Autodesk Inventor part; units mm, degrees
ref_plane "YZ Plane" through (0, 0, 0) normal (1, 0, 0) x (0, 1, 0)
ref_plane "XZ Plane" through (0, 0, 0) normal (0, 1, 0) x (-1, 0, 0)
ref_plane "XY Plane" through (0, 0, 0) normal (0, 0, 1) x (1, 0, 0)
sketch "Эскиз1" plane through (0, 0, 0) normal (0, 1, 0) x (-1, 0, 0)
  circle A0 centre (0, 0) radius 56
  circle A1 centre (46, 0) radius 5.5
  circle A2 centre (0, 46) radius 5.5
  circle A3 centre (-46, 0) radius 5.5
  circle A4 centre (0, -46) radius 5.5
  dimension "d0" = 112
  dimension "d1" = 11
  dimension "d2" = 46
  dimension "d5" = 360
extrude "Выдавливание1" add sketch "Эскиз1" along normal blind 10
sketch "Эскиз3" plane through (0, 10, 0) normal (0, 1, 0) x (1, 0, 0)
  circle A0 centre (0, 0) radius 22
  dimension "d9" = 44
extrude "Выдавливание2" cut sketch "Эскиз3" against normal blind 10
sketch "Эскиз4" plane through (0, 0, 0) normal (0, -1, 0) x (1, 0, 0)
  circle A0 centre (0, 0) radius 38
  dimension "d12" = 76
extrude "Выдавливание3" add sketch "Эскиз4" along normal blind 38
sketch "Эскиз5" plane through (0, -38, 0) normal (0, -1, 0) x (1, 0, 0)
  circle A0 centre (0, 0) radius 12.5
  dimension "d15" = 25
extrude "Выдавливание4" cut sketch "Эскиз5" against normal through all
chamfer "Фаска1" distance 1.6 angle 45 1 edges at (-22, 10, 0)
chamfer "Фаска2" distance 2.5 angle 45 1 edges at (-38, -38, 0)
sketch "Эскиз6" plane through (0, -38, 0) normal (0, -1, 0) x (1, 0, 0)
  point P0 (0, 0)
  point P1 (0, -24)
  point P2 (0, 24)
  dimension "d24" = 24
  dimension "d25" = 48
hole "Отверстие1" at (0, -38, -24) at (0, -38, 24) direction (0, 1, 0) diameter 8.376 depth 24 tip angle 120
chamfer "Фаска3" distance 1.6 angle 45 2 edges at (0, -38, -19.812) (0, -38, 28.188)
properties part number "Фланец"
CAD build for the part. Positions are in the model's coordinates, mm. A direction names the side the tool comes from. Give positions to 0.01 mm unless a question says otherwise; leave off trailing zeros. Order: outer loops, then holes, each group sorted by start corner. A loop starts at its lowest first (then second) coordinate and runs counter-clockwise, first axis right, second up. Notation, with made-up numbers: (19, 62.5) - (31, 62.5) arc R35 ccw to (31, 96.5) - close; hole circle Ø3 at (82, 73.25). An arc over 180 degrees is marked (long way). Answer in a Markdown table with one row per item.
1. Flat gauge pins, fed straight in: pin 1 (10 mm diameter, centred on x = 46, z = 0, fed in from +Y); pin 2 (14.5 mm diameter, centred on x = 0, z = 46, fed in from +Y); pin 3 (8 mm diameter, centred on y = -10.5, z = 1.5, fed in from +X); pin 4 (1.5 mm diameter, centred on x = 24, y = -28.5, fed in from +Z). Where does each tip first touch, or does it go through?
Data:
| item | result |
|---|---|
| pin 1 | passes through |
| pin 2 | stops at y = 10 |
| pin 3 | stops at x = 38 |
| pin 4 | stops at z = 30.06 |
2. Tool access for faces 4 (the flat face through (1, 10, -24)), 5 (the cylindrical face through (-4.769, 4.259, 21.477)), 6 (the flat face through (-37, 0, -12)): list every direction of +Z, -Z, +X, -X, +Y, -Y with a clear straight run to the whole face (end or side of a thin tool).
Data:
| item | result |
|---|---|
| face 4 | +Z, -Z, +X, -X, +Y |
| face 5 | +Y |
| face 6 | -Y |
3. Pull direction X, two halves, no side cores. Call faces 1 (the cylindrical face through (0.716, 4.93, -51.453)), 2 (the flat face through (0, -38, -15)), 3 (the conical face through (34.01, -37.844, -10.71)): pulls with the +X half, pulls with the -X half, needs draft (parallel to the pull), parting line crosses it, or undercut.
Data:
| item | result |
|---|---|
| face 1 | undercut |
| face 2 | needs draft |
| face 3 | parting line crosses it |
4. Saw through at B-B, the plane x = -46. Give the cut face in (y, z).
Data:
| item | result |
|---|---|
| outline | (0, -31.94) - (10, -31.94) - (10, -5.5) - (0, -5.5) - close; (0, 5.5) - (10, 5.5) - (10, 31.94) - (0, 31.94) - close |
5. Saw through at C-C, the plane y = 4.5. Give the cut face in (x, z).
Data:
| item | result |
|---|---|
| outline | circle Ø112 at (0, 0); hole circle Ø11 at (-46, 0); hole circle Ø44 at (0, 0); hole circle Ø11 at (0, -46); hole circle Ø11 at (0, 46); hole circle Ø11 at (46, 0) |
6. Saw through at A-A, the plane z = -44. Give the cut face in (x, y), plus the area to 3 significant figures.
Data:
| item | result |
|---|---|
| outline | (-34.64, 0) - (-5.12, 0) - (-5.12, 10) - (-34.64, 10) - close; (5.12, 0) - (34.64, 0) - (34.64, 10) - (5.12, 10) - close |
| area | 590 mm² |
7. Probe probe 1 along Z at (x, y) = (0, 4); probe 2 along X at (y, z) = (1, 0.5); probe 3 along Z at (x, y) = (0, -31). List the from-to ranges inside material, lowest first. Write a range as [from, to].
Data:
| item | result |
|---|---|
| probe 1 | z = [-56, -51.5], [-40.5, -22], [22, 40.5], [51.5, 56] |
| probe 2 | x = [-56, -51.48], [-40.52, -21.99], [21.99, 40.52], [51.48, 56] |
| probe 3 | z = [-38, -28.19], [-19.81, -12.5], [12.5, 19.81], [28.19, 38] |
8. Saw through at D-D, the plane y = -8.5. Give the cut face in (x, z), plus the area to 3 significant figures.
Data:
| item | result |
|---|---|
| outline | circle Ø76 at (0, 0); hole circle Ø25 at (0, 0) |
| area | 4,050 mm² |
